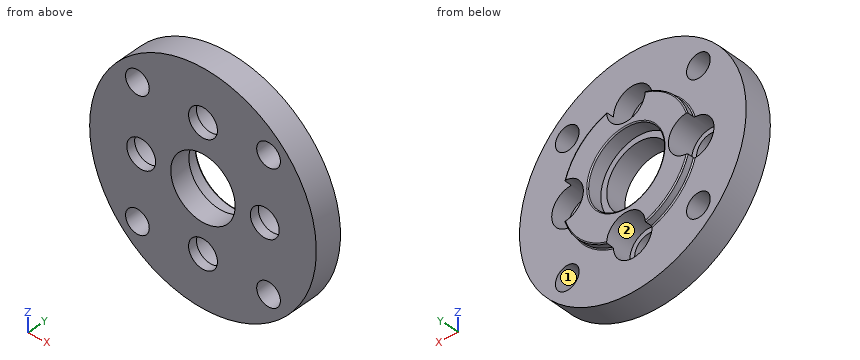
Autodesk Inventor part; units mm, degrees
ref_plane "YZ Plane" through (0, 0, 0) normal (1, 0, 0) x (0, 1, 0)
ref_plane "XZ Plane" through (0, 0, 0) normal (0, 1, 0) x (-1, 0, 0)
ref_plane "XY Plane" through (0, 0, 0) normal (0, 0, 1) x (1, 0, 0)
sketch "Sketch1" plane through (0, 0, 0) normal (0, 1, 0) x (-1, 0, 0)
  circle A0 centre (0, 0) radius 11
  circle A1 centre (0, 0) radius 3.125
  dimension "d0" = 22
  dimension "d1" = 6.25
extrude "Extrusion1" add sketch "Sketch1" along normal blind 2.6
sketch "Sketch2" plane through (0, 2.6, 0) normal (0, 1, 0) x (1, 0, 0)
  circle A0 centre (0, 0) radius 6.25
  circle A1 centre (0, 0) radius 3.125
  dimension "d4" = 12.5
extrude "Extrusion2" add sketch "Sketch2" along normal blind 0.75
sketch "Sketch3" plane through (0, 3.35, 0) normal (0, 1, 0) x (1, 0, 0)
  circle A0 centre (0, 0) radius 3.7
  dimension "d7" = 7.4
extrude "Extrusion3" cut sketch "Sketch3" against normal blind 1.4
sketch "Sketch4" plane through (0, 2.6, 0) normal (0, 1, 0) x (1, 0, 0)
  circle A0 centre (0, 0) radius 11 construction
  line L0 (0, 0) -> (-11, 0)
  circle A1 centre (0, 0) radius 11
  circle A2 centre (-6, 0) radius 1.4
  circle A3 centre (0, -6) radius 1.4
  circle A4 centre (6, 0) radius 1.4
  circle A5 centre (0, 6) radius 1.4
  dimension "d10" = 22
  dimension "d11" = 2.8
  dimension "d12" = 6
  dimension "d15" = 360
extrude "Extrusion4" cut sketch "Sketch4" along normal through all both and the other way through all contours A2 L0 | L0 A2 | A3 | A4 | A5
sketch "Sketch5" plane through (0, 3.35, 0) normal (0, 1, 0) x (1, 0, 0)
  circle A0 centre (-6, 0) radius 1.4
  circle A1 centre (-6, 0) radius 1.875
  circle A2 centre (0, -6) radius 1.875
  circle A3 centre (6, 0) radius 1.875
  circle A4 centre (0, 6) radius 1.875
  point P0 (0, 0)
  dimension "d19" = 3.75
  dimension "d22" = 360
extrude "Extrusion5" cut sketch "Sketch5" against normal blind 2.5 contours A0 | A1 | A2 | A3 | A4
sketch "Sketch6" plane through (0, 2.6, 0) normal (0, 1, 0) x (1, 0, 0)
  line L0 (0, 0) -> (-7.7782, -7.7782) construction
  circle A0 centre (0, 0) radius 11
  line L1 (0, 0) -> (11, 0) construction
  circle A1 centre (0, 0) radius 9 construction
  circle A2 centre (-6.364, -6.364) radius 1.15
  circle A3 centre (6.364, -6.364) radius 1.15
  circle A4 centre (6.364, 6.364) radius 1.15
  circle A5 centre (-6.364, 6.364) radius 1.15
  dimension "d27" = 18
  dimension "d26" = 135
  dimension "d28" = 2.3
  dimension "d31" = 360
extrude "Extrusion6" cut sketch "Sketch6" against normal through all contours A2 | A3 | A4 | A5
fillet "Fillet1" radius 0.1 9 edges at (-3.7, 3.35, 0) (-4.4194, 3.35, 4.4194) (-4.4194, 3.35, -4.4194) (4.4194, 3.35, -4.4194) (4.4194, 3.35, 4.4194) (4.4194, 2.6, 4.4194) (4.4194, 2.6, -4.4194) (-4.4194, 2.6, 4.4194) (-4.4194, 2.6, -4.4194)
properties part number "Motor Plate" material "Aluminum 6061"
Geometry check sheet. Reference: the model listing, model coordinates, mm. Face numbers are marked on the shaded views. A direction names the side the tool comes from. Coordinates: 2 decimals unless noted, no trailing zeros. Write each loop counter-clockwise with the first axis right and the second up, starting at its lowest first coordinate (ties: lowest second). Pieces come first, ordered by that corner, then holes. Notation, with made-up numbers: (33.25, -35.5) -> (82.25, -35.5) arc R15 ccw to (82.25, -28.5) -> close; hole circle Ø6 at (64.5, -35.75). An arc over 180 degrees is marked (long way). Use CSV: the item, a comma, the result in double quotes. Start each with the question number.
Item 1: Thickness scan on line 1 (Z direction, x = 0, y = 1.15) (3 decimals); line 2 (Z direction, x = 0, y = 0.55) (3 decimals); line 3 (X direction, y = 1.95, z = -6.25). Record the ranges inside material, lowest first.
Item 2: Cross-section at D-D, the plane z = 8.5. Record the cut outline in (x, y).
Item 3: Cross-section at A-A, the plane z = 0. State how many separate pieces and enclosed holes the cut face has, plus the area to 3 significant figures.
Item 4: Set-up check for the marked faces 1 and 2: record each of +Z, -Z, +X, -X, +Y, -Y from which the full face is reachable in a straight line by a thin tool's end or side.
Item 5: Depth check by flat-ended pin: pin 1 Ø2 at (x, y) = (8.5, 3) entering from -Z; pin 2 Ø2 at (y, z) = (1, -3) entering from +X; pin 3 Ø1.5 at (x, y) = (-8.5, 2.5) entering from +Z. Enter the tip coordinate at first touch or a pass-through.
Answers:
1,line 1,"-11 to -7.875, -4.125 to -3.125, 3.125 to 4.125, 7.875 to 11"
1,line 2,"-11 to -7.4, -4.6 to -3.125, 3.125 to 4.6, 7.4 to 11"
1,line 3,"-9.05 to -7.51, -5.22 to -1.86, 1.86 to 5.22, 7.51 to 9.05"
2,outline,"(-6.98, 0) -> (6.98, 0) -> (6.98, 2.6) -> (-6.98, 2.6) -> close"
3,separate pieces,"4"
3,enclosed holes,"0"
3,area,"23.0 mm^2"
4,face 1,"+Y, -Y"
4,face 2,"+Y"
5,pin 1,"z = -7.97"
5,pin 2,"x = 10.82"
5,pin 3,"z = 7.81"
